Autodesk Inventor part; units mm, degrees
ref_plane "YZ Plane" through (0, 0, 0) normal (1, 0, 0) x (0, 1, 0)
ref_plane "XZ Plane" through (0, 0, 0) normal (0, 1, 0) x (-1, 0, 0)
ref_plane "XY Plane" through (0, 0, 0) normal (0, 0, 1) x (1, 0, 0)
sketch "Sketch1" plane through (0, 0, 0) normal (1, 0, 0) x (0, 1, 0)
  circle A0 centre (0, 0) radius 14.2875
  circle A1 centre (0, -177.8) radius 14.2875
  line L0 (152.4, -31.75) -> (-152.4, -31.75) construction
  line L1 (-152.4, -31.75) -> (-152.4, -146.05) construction
  line L2 (-152.4, -146.05) -> (152.4, -146.05) construction
  line L3 (152.4, -146.05) -> (152.4, -31.75) construction
  line L4 (152.4, -31.75) -> (-152.4, -146.05) construction
  line L5 (-152.4, -31.75) -> (152.4, -146.05) construction
  circle A2 centre (0, 0) radius 38.1 construction
  circle A3 centre (0, -177.8) radius 38.1 construction
  circle A4 centre (0, 0) radius 31.75 construction
  circle A5 centre (0, -177.8) radius 31.75 construction
  circle A6 centre (0, 0) radius 26.9875 construction
  circle A7 centre (0, -177.8) radius 26.9875 construction
  circle A8 centre (97.4242, -177.8) radius 14.2875
  circle A9 centre (97.4242, -177.8) radius 38.1 construction
  circle A10 centre (97.4242, -177.8) radius 31.75 construction
  circle A11 centre (97.4242, -177.8) radius 26.9875 construction
  circle A12 centre (97.4242, 0) radius 14.2875
  circle A13 centre (97.4242, 0) radius 38.1 construction
  circle A14 centre (97.4242, 0) radius 31.75 construction
  circle A15 centre (97.4242, 0) radius 26.9875 construction
  line L6 (97.4242, -204.7875) -> (0, -204.7875)
  line L7 (97.4242, 26.9875) -> (0, 26.9875)
  line L8 (124.4117, 0) -> (124.4117, -177.8)
  line L9 (-26.9875, 0) -> (-26.9875, -177.8)
  arc A16 (124.4117, 0) -> (97.4242, 26.9875) centre (97.4242, 0) ccw
  arc A17 (97.4242, -204.7875) -> (124.4117, -177.8) centre (97.4242, -177.8) ccw
  arc A18 (0, 26.9875) -> (-26.9875, 0) centre (0, 0) ccw
  arc A19 (-26.9875, -177.8) -> (0, -204.7875) centre (0, -177.8) ccw
  line L10 (97.4242, -177.8) -> (0, -177.8) construction
  circle A20 centre (81.6238, -143.1307) radius 14.2875
  circle A21 centre (97.4242, -177.8) radius 19.05 construction
  circle A22 centre (81.6238, -143.1307) radius 19.05 construction
  point P0 (0, -88.9)
  point P1 (48.7121, 0)
  point P2 (48.7121, -177.8)
  point P3 (48.7121, -177.8)
  dimension "d0" = 28.575
  dimension "d2" = 304.8
  dimension "d3" = 114.3
  dimension "d4" = 76.2
  dimension "d6" = 6.35
  dimension "d7" = 12.7
  dimension "d8" = 97.4242
  dimension "d38" = 177.8
  dimension "d40" = 38.1
  dimension "d41" = 144.0002
extrude "Extrusion1" add sketch "Sketch1" along normal blind 6.35 contours L6 A19 L9 A18 L7 A16 L8 A17 | A20
hole "Hole1" at (0, 48.7121, 0) at (0, 48.7121, -177.8) direction (1, 0, 0) diameter 5.1054 end through all
sketch "Sketch3" plane through (6.35, 0, 0) normal (1, 0, 0) x (0, 0, -1)
  line L0 (-26.9875, 97.4242) -> (-26.9875, 0) construction
  line L1 (0, -26.9875) -> (177.8, -26.9875) construction
  point P0 (0, 0)
  point P1 (-20.6375, 36.5125)
  dimension "d29" = 6.35
  dimension "d30" = 63.5
hole "Hole2" at (6.35, 36.5125, 20.6375) direction (-1, 0, 0) diameter 3.302 end through all
extrude "Extrusion2" cut sketch "Sketch1" along normal through all contours A20
equation "\"d36\" = Thickness"
equation "\"BendRadius\" = Thickness"
equation "\"BendReliefWidth\" = Thickness"
equation "\"BendReliefDepth\" = 0.5 * Thickness"
equation "\"CornerReliefSize\" = 4 * Thickness"
equation "\"MinimumRemnant\" = 2 * Thickness"
equation "\"TransitionRadius\" = BendRadius"
equation "\"JacobiRadiusSize\" = BendRadius"
equation "\"GapSize\" = Thickness"
equation "\"d18\" = Thickness"
properties part number "GP4-006" material "Polycarbonate, Smoke"
The listing builds one solid part. Answer for the finished solid, in the listing's coordinates (mm). Coordinates: 2 decimals unless noted, no trailing zeros. Order: outer loops, then holes, each group sorted by start corner. A loop starts at its lowest first (then second) coordinate and runs counter-clockwise, first axis right, second up. Notation, with made-up numbers: M -17.75,84 L -13.75,84 A26 cw -13.75,113 Z; hole C -7,17 d6. An arc over 180 degrees is marked long. Use CSV: the item, a comma, the result in double quotes.
Q1. Section D-D (x = 3) is taken. Give the number of separate pieces and of enclosed holes in the cut face, then the cut area to 3 significant figures.
Here are the results:
separate pieces,"1"
enclosed holes,"8"
area,"31,200 mm2"
Q2. Section B-B (z = -187.5) is taken. Determine the outline of the cut face in (x, y).
Here are the results:
outline,"M 0,-25.18 L 6.35,-25.18 L 6.35,-10.49 L 0,-10.49 Z; M 0,10.49 L 6.35,10.49 L 6.35,86.93 L 0,86.93 Z; M 0,107.91 L 6.35,107.91 L 6.35,122.61 L 0,122.61 Z"
Q3. Section C-C (y = 11) is taken. Determine the outline of the cut face in (x, z), then the cut area to 3 significant figures.
Here are the results:
outline,"M 0,-204.79 L 6.35,-204.79 L 6.35,-186.92 L 0,-186.92 Z; M 0,-168.68 L 6.35,-168.68 L 6.35,-9.12 L 0,-9.12 Z; M 0,9.12 L 6.35,9.12 L 6.35,26.99 L 0,26.99 Z"
area,"1,240 mm2"
Q4. Straight lines are drawn through the part: L1, parallel to Z at x = 1.5, y = 0; L2, parallel to Z at x = 1, y = 11.5; L3, parallel to Y at x = 4.75, z = -185. For each, find the intervals that lie inside material, in ascending order.
Here are the results:
L1,"-204.79 to -192.09, -163.51 to -14.29, 14.29 to 26.99"
L2,"-204.79 to -186.28, -169.32 to -8.48, 8.48 to 26.99"
L3,"-26.01 to -12.34, 12.34 to 85.08, 109.76 to 123.43"
Q5. Determine the mould class of faces 1 (the flat face through (3, 124.412, -88)), 2 (the flat face through (3, 49, 26.988)), 3 (the cylindrical face through (3.131, -1.86, -191.966)), 4 (the cylindrical face through (3.131, -18.872, -197.092)) for opening direction Y: pulls with the +Y half, pulls with the -Y half, needs draft (parallel to the pull), parting line crosses it, or undercut.
Here are the results:
face 1,"pulls with the +Y half"
face 2,"needs draft"
face 3,"undercut"
face 4,"pulls with the -Y half"
Q6. Section A-A (z = -154) is taken. Determine the outline of the cut face in (x, y), then the cut area to 3 significant figures.
Here are the results:
outline,"M 0,-26.99 L 6.35,-26.99 L 6.35,72.35 L 0,72.35 Z; M 0,90.9 L 6.35,90.9 L 6.35,124.41 L 0,124.41 Z"
area,"844 mm2"
Q7. Given pin 1 Ø6 at (y, z) = (48.71, 0) entering from +X; pin 2 Ø3 at (y, z) = (48.71, -177.8) entering from -X; pin 3 Ø1 at (x, y) = (3.5, -3.5) entering from -Z, each flat-ended and moving along its own axis, determine where each tip first touches the part or whether it passes through.
Here are the results:
pin 1,"x = 6.35"
pin 2,"through"
pin 3,"z = -204.62"
